For this review, take the finished solid that the model builds, in its own axes (mm). Face numbers are marked on the shaded views. A direction names the side the tool comes from. Round coordinates to 2 decimals unless told otherwise and drop trailing zeros. Write each loop counter-clockwise with the first axis right and the second up, starting at its lowest first coordinate (ties: lowest second). Pieces come first, ordered by that corner, then holes. Notation, with made-up numbers: (58.5, 77.25) -> (99.5, 77.25) arc R20 cw to (99.5, 106.25) -> close; hole circle Ø11 at (-6, -13). An arc over 180 degrees is marked (long way). Answer in a Markdown table with one row per item.
Autodesk Inventor part; units mm, degrees
ref_plane "YZ Plane" through (0, 0, 0) normal (1, 0, 0) x (0, 1, 0)
ref_plane "XZ Plane" through (0, 0, 0) normal (0, 1, 0) x (-1, 0, 0)
ref_plane "XY Plane" through (0, 0, 0) normal (0, 0, 1) x (1, 0, 0)
sketch "Skizze1" plane through (0, 0, 0) normal (0, 0, 1) x (1, 0, 0)
  circle A0 centre (17.75, 57) radius 2.15
  circle A1 centre (62.75, 57) radius 2.15
  circle A2 centre (17.75, 17) radius 2.15
  circle A3 centre (62.75, 17) radius 2.15
  line L0 (70.5, 64) -> (10, 64)
  line L1 (10, 64) -> (10, -3)
  line L2 (70.5, -3) -> (70.5, 64)
  line L3 (10, -3) -> (70.5, -3)
  line L4 (0, 0) -> (0, 8)
  line L5 (0, 8) -> (-15, 8)
  line L6 (-15, -8) -> (-15, 8)
  line L7 (0, -8) -> (-15, -8)
  line L8 (70.5, -8) -> (70.5, 64)
  line L9 (10, 64) -> (10, 8)
  line L10 (-15, 8) -> (10, 8)
  line L11 (70.5, -8) -> (-15, -8)
  line L12 (-15, 8) -> (-15, -8)
  point P0 (-10, 0)
  dimension "d0" = 16
extrude "Extrusion1" add sketch "Skizze1" along normal blind 10
properties part number "Seiten_Platte"
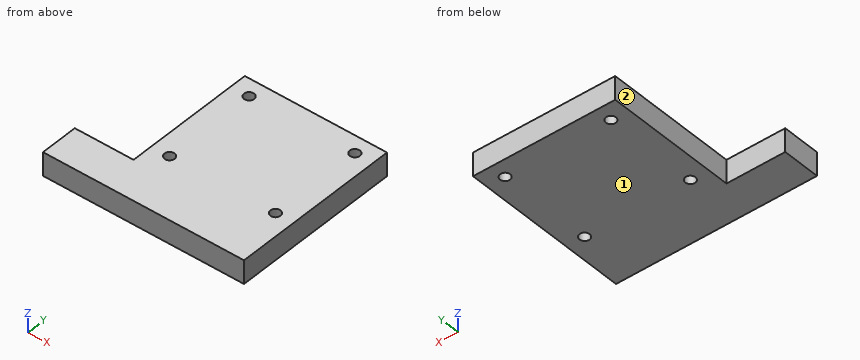
1) Consider section B-B on x = 62.75. State the section outline as (y, z) points.
Solved:
| item | result |
|---|---|
| outline | (-8, 0) -> (14.85, 0) -> (14.85, 10) -> (-8, 10) -> close; (19.15, 0) -> (54.85, 0) -> (54.85, 10) -> (19.15, 10) -> close; (59.15, 0) -> (64, 0) -> (64, 10) -> (59.15, 10) -> close |
2) Consider section C-C on z = 6.75. State the section outline as (x, y) points.
Solved:
| item | result |
|---|---|
| outline | (-15, -8) -> (70.5, -8) -> (70.5, 64) -> (10, 64) -> (10, 8) -> (-15, 8) -> close; hole circle Ø4.3 at (17.75, 17); hole circle Ø4.3 at (17.75, 57); hole circle Ø4.3 at (62.75, 17); hole circle Ø4.3 at (62.75, 57) |
3) Consider section A-A on y = 57. State the section outline as (x, z) points, then the cut area to 3 significant figures.
Solved:
| item | result |
|---|---|
| outline | (10, 0) -> (15.6, 0) -> (15.6, 10) -> (10, 10) -> close; (19.9, 0) -> (60.6, 0) -> (60.6, 10) -> (19.9, 10) -> close; (64.9, 0) -> (70.5, 0) -> (70.5, 10) -> (64.9, 10) -> close |
| area | 519 mm² |
4) Clearance check with flat-ended pins moving along their axes: pin 1 Ø5 at (x, y) = (17.75, 17) entering from -Z; pin 2 Ø2 at (y, z) = (12.5, 3) entering from -X; pin 3 Ø3 at (x, z) = (0, 6) entering from +Y. State where each tip first meets the part, or that it passes through.
Solved:
| item | result |
|---|---|
| pin 1 | z = 0 |
| pin 2 | x = 10 |
| pin 3 | y = 8 |
5) Consider section D-D on y = 23.5. State the section outline as (x, z) points, then the cut area to 3 significant figures.
Solved:
| item | result |
|---|---|
| outline | (10, 0) -> (70.5, 0) -> (70.5, 10) -> (10, 10) -> close |
| area | 605 mm² |
6) For line 1 (Y direction, x = 17.75, z = 7); line 2 (Y direction, x = 6, z = 4.5); line 3 (X direction, y = 25.5, z = 9.25), list the stretches that pass through material, from the lowest coordinate up. Write a range as [from, to].
Solved:
| item | result |
|---|---|
| line 1 | [-8, 14.85], [19.15, 54.85], [59.15, 64] |
| line 2 | [-8, 8] |
| line 3 | [10, 70.5] |
7) For the marked faces 1 and 2, list the 3-axis set-ups (+Z, -Z, +X, -X, +Y, -Y) from which the entire face can be reached by the end or side of a thin tool; tool diameter is ignored.
Solved:
| item | result |
|---|---|
| face 1 | -Z, +X, -X, +Y, -Y |
| face 2 | +Z, -Z, -X, +Y |
